Here's how the part is built. I have some questions about the finished solid (model axes, mm). A direction names the side the tool comes from. Round coordinates to 2 decimals unless told otherwise and drop trailing zeros. Loops run counter-clockwise (first coordinate to the right, second up) from the corner with the lowest first, then second, coordinate; pieces in that order, holes last. Notation, with made-up numbers: M 5,77 L 32,77 A20 ccw 32,114 Z; hole C 64,-14 d10. An arc over 180 degrees is marked long. Answer as a JSON object with one key per item and string values.
Autodesk Inventor part; units mm, degrees
ref_plane "YZ Plane" through (0, 0, 0) normal (1, 0, 0) x (0, 1, 0)
ref_plane "XZ Plane" through (0, 0, 0) normal (0, 1, 0) x (-1, 0, 0)
ref_plane "XY Plane" through (0, 0, 0) normal (0, 0, 1) x (1, 0, 0)
sketch "Esboço1" plane through (0, 0, 0) normal (0, 1, 0) x (-1, 0, 0)
  line L0 (0, 0) -> (80, 0)
  line L1 (80, -170) -> (0, -170)
  line L2 (80, -40) -> (0, -40)
  line L3 (0, -40) -> (0, -100)
  line L4 (0, -100) -> (80, -100)
  line L5 (80, -100) -> (80, -40)
  line L6 (80, 0) -> (80, -35)
  line L7 (80, -35) -> (90, -35)
  line L8 (90, -35) -> (90, -105)
  line L9 (80, 0) -> (80, -35)
  line L10 (80, -40) -> (80, -100)
  line L11 (90, -70) -> (0, -70)
  line L12 (40, 0) -> (40, -170)
  line L13 (0, -35) -> (-10, -35)
  line L14 (-10, -35) -> (-10, -105)
  line L15 (0, -35) -> (0, 0)
  line L16 (0, -100) -> (0, -40)
  line L17 (52.5, -114) -> (27.5, -114)
  line L18 (27.5, -114) -> (27.5, -151)
  line L19 (27.5, -151) -> (52.5, -151)
  line L20 (52.5, -151) -> (52.5, -114)
  line L21 (82, -38) -> (-2, -38)
  line L22 (-2, -102) -> (82, -102)
  circle A0 centre (84.5595, -70) radius 1.75
  line L23 (84.5595, -66.5) -> (82, -66.5)
  line L24 (82, -73.5) -> (84.5595, -73.5)
  arc A1 (84.5595, -73.5) -> (84.5595, -66.5) centre (83.9005, -70) ccw
  line L25 (82, -102) -> (82, -73.5)
  line L26 (82, -66.5) -> (82, -38)
  circle A2 centre (-4.5595, -70) radius 1.75
  line L27 (-4.5595, -66.5) -> (-2, -66.5)
  line L28 (-2, -73.5) -> (-4.5595, -73.5)
  arc A3 (-4.5595, -66.5) -> (-4.5595, -73.5) centre (-3.9005, -70) ccw
  line L29 (-2, -38) -> (-2, -66.5)
  line L30 (-2, -73.5) -> (-2, -102)
  line L31 (90, -105) -> (90, -151)
  line L32 (90, -151) -> (90, -170)
  line L33 (90, -170) -> (-10, -170)
  line L34 (-10, -170) -> (-10, -105)
  line L35 (80, -35) -> (0, -35)
  circle A4 centre (-3, -120) radius 1.75
  circle A5 centre (83, -120) radius 1.75
  circle A6 centre (7, -7) radius 1.5
  circle A7 centre (73, -7) radius 1.5
  line L36 (52.5, -114) -> (60.5, -114)
  line L37 (60.5, -114) -> (60.5, -151)
  line L38 (60.5, -151) -> (52.5, -151)
  line L39 (52.5, -151) -> (52.5, -114)
  circle A8 centre (56.5, -120) radius 1.75
  circle A9 centre (56.5, -145) radius 1.75
  line L40 (27.5, -114) -> (19.5, -114)
  line L41 (19.5, -114) -> (19.5, -151)
  line L42 (19.5, -151) -> (27.5, -151)
  circle A10 centre (23.5, -120) radius 1.75
  circle A11 centre (23.5, -145) radius 1.75
  point P0 (45, -70)
  point P1 (40, -102)
  point P2 (80, -17.5)
  point P3 (0, -170)
  point P4 (56.5, -114)
  point P5 (56.5, -151)
  dimension "d3" = 60
  dimension "d4" = 35
  dimension "d5" = 10
  dimension "d6" = 70
  dimension "d7" = 30
  dimension "d9" = 80
  dimension "d12" = 64
  dimension "d13" = 32
  dimension "d15" = 3.5
  dimension "d16" = 3.5
  dimension "d17" = 37
  dimension "d18" = 25
  dimension "d19" = 12.5
  dimension "d21" = 19
  dimension "d22" = 12
  dimension "d23" = 80
  dimension "d30" = 3.5
  dimension "d31" = 7
  dimension "d32" = 50
  dimension "d33" = 3
  dimension "d35" = 3.5
  dimension "d36" = 7
  dimension "d37" = 7
  dimension "d54" = 8
  dimension "d55" = 3.5
  dimension "d56" = 3.5
  dimension "d57" = 6
  dimension "d58" = 6
  dimension "d59" = 4
  dimension "d60" = 4
  dimension "d63" = 135
extrude "Extrusão1" add sketch "Esboço1" along normal blind 23 contours L21 L26 L23 A1 L11 A0 L5 L2 L12 | L12 L2 L3 L4 L22 L30 L28 A3 L27 L29 L21 | A1 L24 L25 L22 L12 L4 L5 L11 A0
extrude "Extrusão4" add sketch "Esboço1" along normal blind 2.5 contours L0 L12 L35 L15 | L0 L6 L35 L12
extrude "Extrusão5" add sketch "Esboço1" along normal blind 5 contours L35 L12 L21 L29 L27 A3 L28 L30 L22 L17 L40 L41 L42 L19 L1 L33 L34 L14 L13 | L35 L7 L8 L11 A1 L23 L26 L21 L12 | L12 L11 L3 L2 | L2 L5 L11 L12 | L8 L31 L32 L33 L1 L12 L19 L38 L37 L36 L17 L22 L25 L24 A1 L11 | L12 L4 L3 L11 | L11 L5 L4 L12 | L42 L41 L40 L18 | L20 L36 L37 L38 | A8 | A9 | A10 | A11
chamfer "Chanfro1" distance 2.5 angle 45 1 edges at (-40, 5, -102)
chamfer "Chanfro2" distance 2.5 angle 45 4 edges at (2, 5, -87.75) (7.462, 5, -70) (3.2797, 5, -73.5) (2, 5, -52.25)
chamfer "Chanfro3" distance 2.5 angle 45 1 edges at (4.5297, 5, -66.5)
chamfer "Chanfro4" distance 2.5 angle 45 5 edges at (-82, 5, -87.75) (-87.462, 5, -70) (-82, 5, -52.25) (-83.2797, 5, -73.5) (-83.2797, 5, -66.5)
extrude "Extrusão6" cut sketch "Esboço1" along normal mid plane 10 contours A8 | A9 | A10 | A11
properties part number "peca_principal"
Item 1: I want a section at D-D, the plane z = -70. State how many separate pieces and enclosed holes the cut face has, then the cut area to 3 significant figures.
Resolved:
{"separate pieces": "3", "enclosed holes": "0", "area": "614 mm²"}
Item 2: I want a section at A-A, the plane z = -120. Please give me the cut outline in (x, y).
Resolved:
{"outline": "M -90,0 L -84.75,0 L -84.75,5 L -90,5 Z; M -81.25,0 L -58.25,0 L -58.25,5 L -81.25,5 Z; M -54.75,0 L -52.5,0 L -52.5,5 L -54.75,5 Z; M -27.5,0 L -25.25,0 L -25.25,5 L -27.5,5 Z; M -21.75,0 L 1.25,0 L 1.25,5 L -21.75,5 Z; M 4.75,0 L 10,0 L 10,5 L 4.75,5 Z"}
Item 3: I want a section at C-C, the plane y = 19. Please give me the cut outline in (x, z).
Resolved:
{"outline": "M -84.56,-73.5 L -82,-73.5 L -82,-102 L 2,-102 L 2,-73.5 L 4.56,-73.5 A3.56 ccw 4.56,-66.5 L 2,-66.5 L 2,-38 L -82,-38 L -82,-66.5 L -84.56,-66.5 A3.56 ccw Z; hole C -84.56,-70 d3.5; hole M -80,-100 L 0,-100 L 0,-40 L -80,-40 Z; hole C 4.56,-70 d3.5"}
Item 4: Please list where these lines run through material, in increasing order: probe 1 along Z at (x, y) = (-56.5, 3.05); probe 2 along X at (y, z) = (18, -70); probe 3 along X at (y, z) = (1.45, -120). Write a range as from..to.
Resolved:
{"probe 1": "-170..-146.75, -143.25..-121.75, -118.25..-35", "probe 2": "-87.46..-86.31, -82.81..-80, 0..2.81, 6.31..7.46", "probe 3": "-90..-84.75, -81.25..-58.25, -54.75..-52.5, -27.5..-25.25, -21.75..1.25, 4.75..10"}
Item 5: I want a section at B-B, the plane x = -56.5. Please give me the cut outline in (y, z).
Resolved:
{"outline": "M 0,-170 L 5,-170 L 5,-146.75 L 0,-146.75 Z; M 0,-143.25 L 5,-143.25 L 5,-121.75 L 0,-121.75 Z; M 0,-118.25 L 5,-118.25 L 5,-104.5 L 7.5,-102 L 23,-102 L 23,-100 L 5,-100 L 5,-40 L 23,-40 L 23,-38 L 5,-38 L 5,-35 L 2.5,-35 L 2.5,0 L 0,0 Z"}
Item 6: I'm going to push flat-ended pins straight in: pin 1 Ø3 at (x, y) = (3, 13) entering from +Z; pin 2 Ø12 at (y, z) = (14.5, -101) entering from -X; pin 3 Ø4 at (x, y) = (-58, 20) entering from -Z. Where does each tip first touch, or does it pass through?
Resolved:
{"pin 1": "z = -38", "pin 2": "x = -82", "pin 3": "z = -102"}
Item 7: On a 3-axis mill with a long thin cutter (end or side, diameter ignored), from which of +Z, -Z, +X, -X, +Y, -Y can I reach the whole of each face in a straight line? I mean faces 1 (the face through (2, 15, -88)), 2 (the face through (-41, 14, -38)), 3 (the face through (-80, 14, -70)), 4 (the face through (2, 15, -52)). Say none if no direction works.
Resolved:
{"face 1": "-Z, +X, +Y", "face 2": "+Z, +X, -X, +Y", "face 3": "+Y", "face 4": "+Z, +X, +Y"}
Item 8: If we mould it in two halves opening along Z, with no side actions, what happens to faces 5 (the face through (-40, 2, -151)), 6 (the face through (7.46, 15.14, -70.07)), 7 (the face through (-39, 15, -102))? For each: pulls with the +Z half, pulls with the -Z half, needs draft (parallel to the pull), parting line crosses it, or undercut.
Resolved:
{"face 5": "undercut", "face 6": "parting line crosses it", "face 7": "pulls with the -Z half"}
